Design review of the part built by this model. Coordinates are the model's own, in mm. A direction names the side the tool comes from. Coordinates: 2 decimals unless noted, no trailing zeros. Write each loop counter-clockwise with the first axis right and the second up, starting at its lowest first coordinate (ties: lowest second). Pieces come first, ordered by that corner, then holes. Notation, with made-up numbers: M -19.75,13.5 L 38.25,13.5 A22 ccw 38.25,34.5 Z; hole C 80,1.5 d6. An arc over 180 degrees is marked long. Return JSON: item names as keys, results as strings. Group by question number.
```python
from build123d import *

# Parameters (mm, degrees)
SKETCH1_W                   = 39.6875
SKETCH1_H                   = 31.75
BOSS_EXTRUDE1_DEPTH         = 6.35
SKETCH2_R                   = 3.175
CUT_EXTRUDE1_DEPTH          = 6.35
CUT_EXTRUDE4_DEPTH          = 6.35
SKETCH4_W                   = 12.7
SKETCH4_H                   = 6.35
SKETCH4_R                   = 1.7526
BOSS_EXTRUDE2_DEPTH         = 6.35
SKETCH5_R                   = 6.35
CUT_EXTRUDE3_DEPTH          = 6.35
TAP_DRILL_FOR_M3X0_5_TAP1_D = 2.5


with BuildPart() as part:
    # Sketch1 → Boss-Extrude1 (new body)
    with BuildSketch(Plane.XY):
        with Locations((-19.84375, 0)):
            Rectangle(SKETCH1_W, SKETCH1_H)
    boss_extrude1 = extrude(amount=BOSS_EXTRUDE1_DEPTH)

    # Sketch2 → Cut-Extrude1 (cut)
    with BuildSketch(Plane.XY.offset(6.35)):
        with Locations((-19.05, 0)):
            Circle(SKETCH2_R)
    extrude(amount=-CUT_EXTRUDE1_DEPTH, mode=Mode.SUBTRACT)

    # Sketch3 → Cut-Extrude4 (cut)
    with BuildSketch(Plane.XY.offset(6.35)):
        Polygon((-35.23615, 6.096), (-31.43885, 6.096), (-31.43885, 9.5964375), (-29.36875, 9.5964375), (-29.36875, 12.3745625), (-31.43885, 12.3745625), (-31.43885, 15.875), (-35.23615, 15.875), (-35.23615, 12.3745625), (-37.30625, 12.3745625), (-37.30625, 9.5964375), (-35.23615, 9.5964375), align=None)
    cut_extrude4 = extrude(amount=-CUT_EXTRUDE4_DEPTH, mode=Mode.SUBTRACT)

    # Sketch4 → Boss-Extrude2 (add)
    with BuildSketch(Plane.XY.offset(6.35)):
        with Locations((-19.84375, 19.05)):
            Rectangle(SKETCH4_W, SKETCH4_H)
        with Locations((-19.84375, 19.05)):
            Circle(SKETCH4_R, mode=Mode.SUBTRACT)
    boss_extrude2 = extrude(amount=-BOSS_EXTRUDE2_DEPTH)

    # Mirror1: Boss-Extrude1, Cut-Extrude4, Boss-Extrude2 across plane
    add(boss_extrude1.mirror(Plane(origin=(0, -15.875, 6.35), x_dir=(0, 0, 1), z_dir=(-1, 0, 0))))
    add(cut_extrude4.mirror(Plane(origin=(0, -15.875, 6.35), x_dir=(0, 0, 1), z_dir=(-1, 0, 0))), mode=Mode.SUBTRACT)
    add(boss_extrude2.mirror(Plane(origin=(0, -15.875, 6.35), x_dir=(0, 0, 1), z_dir=(-1, 0, 0))))

    # Sketch5 → Cut-Extrude3 (cut)
    with BuildSketch(Plane.XY.offset(6.35)):
        with Locations((19.05, 0)):
            Circle(SKETCH5_R)
    extrude(amount=-CUT_EXTRUDE3_DEPTH, mode=Mode.SUBTRACT)

    # Tap Drill for M3x0.5 Tap1 (through all)
    with Locations(Plane.XY.offset(6.35)):
        with Locations((28.05, 0), (10.05, 0)):
            Hole(TAP_DRILL_FOR_M3X0_5_TAP1_D / 2)


solid = part.part
```
Item 1: The part is to be moulded in two halves that separate along X. For faces 5 (the flat face through (29, 15.875, 3)), 6 (the flat face through (-39.688, 0, 3)), 7 (the flat face through (-33, 6.096, 3)), say which applies: pulls with the +X half, pulls with the -X half, needs draft (parallel to the pull), parting line crosses it, or undercut.
Item 2: For line 1 (X direction, y = 5.5, z = 2.25); line 2 (Y direction, x = -30, z = 3) (3 decimals); line 3 (X direction, y = 17, z = 0.5), list the stretches that pass through material, from the lowest coordinate up.
Item 3: Add section C-C (y = 19.05). Write out the cut boundary in (x, z).
Item 4: Add section B-B (y = 0). Count the separate pieces of the cut face and the enclosed holes in it, plus the area to 3 significant figures.
Item 5: Add section D-D (x = 28.05). Write out the cut boundary in (y, z) (3 decimals).
Item 6: For pin 1 (2 mm diameter, centred on x = 38.5, z = 4.5, fed in from +Y) (3 decimals); pin 2 (1.1 mm diameter, centred on x = -33.5, z = 3, fed in from +Y), all flat-tipped, find the tip position at first contact; note any pin that passes through.
Item 7: Add section A-A (y = 8). Write out the cut boundary in (x, z).
Item 8: Machinability: for faces 1 (the flat face through (-31.439, 8, 3)), 2 (the flat face through (37.306, 11, 3)), 3 (the flat face through (-37, 15.875, 3)), 4 (the flat face through (-20, 22.225, 3)), which of the approach directions +Z, -Z, +X, -X, +Y, -Y give a long, thin tool a straight path to every point of the face, cutting with its end or side? Answer none if there is none.
Geometry check:
{
 "1": {"face 5": "needs draft", "face 6": "pulls with the -X half", "face 7": "undercut"},
 "2": {"line 1": "-39.69 to 15.88, 22.22 to 39.69", "line 2": "-15.875 to 9.596, 12.375 to 15.875", "line 3": "-26.19 to -13.49, 13.49 to 26.19"},
 "3": {"outline": "M -26.19,0 L -21.6,0 L -21.6,6.35 L -26.19,6.35 Z; M -18.09,0 L -13.49,0 L -13.49,6.35 L -18.09,6.35 Z; M 13.49,0 L 18.09,0 L 18.09,6.35 L 13.49,6.35 Z; M 21.6,0 L 26.19,0 L 26.19,6.35 L 21.6,6.35 Z"},
 "4": {"separate pieces": "5", "enclosed holes": "0", "area": "351 mm^2"},
 "5": {"outline": "M -15.875,0 L -1.25,0 L -1.25,6.35 L -15.875,6.35 Z; M 1.25,0 L 15.875,0 L 15.875,6.35 L 1.25,6.35 Z"},
 "6": {"pin 1": "y = 15.875", "pin 2": "y = 6.1"},
 "7": {"outline": "M -39.69,0 L -35.24,0 L -35.24,6.35 L -39.69,6.35 Z; M -31.44,0 L 31.44,0 L 31.44,6.35 L -31.44,6.35 Z; M 35.24,0 L 39.69,0 L 39.69,6.35 L 35.24,6.35 Z"},
 "8": {"face 1": "+Z, -Z, +Y", "face 2": "+Z, -Z", "face 3": "+Z, -Z, -X, +Y", "face 4": "+Z, -Z, +X, -X, +Y"}
}
